Part model, mm, in its own coordinate system. A direction names the side the tool comes from. Give positions to 0.01 mm unless a question says otherwise; leave off trailing zeros. Write each loop counter-clockwise with the first axis right and the second up, starting at its lowest first coordinate (ties: lowest second). Pieces come first, ordered by that corner, then holes. Notation, with made-up numbers: M 79.5,48.5 L 96.5,48.5 A33 ccw 96.5,82.5 Z; hole C -20,25.25 d1. An arc over 180 degrees is marked long. Answer as CSV lines item,"result". Start each with the question number.
Item 1: Band-saw the part on C-C, the plane z = -8. List the corners of the cut face in (x, y), then the cut area to 3 significant figures.
Item 2: Pin check, flat tips, straight feed: pin 1 (5 mm diameter, centred on x = 7, z = 5, fed in from +Y); pin 2 (8 mm diameter, centred on x = 7, y = 11.8, fed in from +Z). Stop position of each tip, or through.
Item 3: Wall check: L1, parallel to Y at x = 7, z = -16.25; L2, parallel to Y at x = 8, z = 3; L3, parallel to Z at x = 11.5, y = 8. Give the ranges that are in metal, low to high. Write a range as from..to.
Item 4: Band-saw the part on D-D, the plane x = 13. List the corners of the cut face in (y, z), then the cut area to 3 significant figures.
Item 5: 3-axis set-ups, long thin cutter, end or side, ignore diameter. For faces 5 (the flat face through (7, 20, -15.506)), 6 (the cylindrical face through (8.61, 33.83, -16.49)): which of +Z, -Z, +X, -X, +Y, -Y reach the whole face in a straight line?
Item 6: Two-plate mould, pull along X, no slides. Class faces 1 (the flat face through (14, 1, -7)), 2 (the cylindrical face through (5.851, 1.014, 16.565)), 3 (the flat face through (0, 1, -7)), 4 (the flat face through (7, 0, 2)): +X half, -X half, draft (parallel to the pull), parting line (faces both ways), or undercut.
Item 7: Band-saw the part on B-B, the plane y = 29.5. List the corners of the cut face in (x, z), then the cut area to 3 significant figures.
Item 8: Band-saw the part on A-A, the plane x = 7. List the corners of the cut face in (y, z).
from build123d import *

# Parameters (mm, degrees)
BOSS_EXTRUDE1_DEPTH = 14
SKETCH2_R           = 3
CUT_EXTRUDE1_DEPTH  = 46.02225292
SKETCH3_R           = 3
CUT_EXTRUDE2_DEPTH  = 56.551777649


with BuildPart() as part:
    # Sketch1 → Boss-Extrude1 (new body)
    with BuildSketch(Plane(origin=(0, 0, 0), x_dir=(0, 0, -1), z_dir=(1, 0, 0))):
        Polygon((-21.494261048, 2), (15.505738952, 2), (15.505738952, 39), (17.505738952, 39), (17.505738952, 0), (-21.494261048, 0), align=None)
    extrude(amount=BOSS_EXTRUDE1_DEPTH)

    # Sketch2 → Cut-Extrude1 (cut, through all)
    with BuildSketch(Plane(origin=(0, 2, 0), x_dir=(1, 0, 0), z_dir=(0, 1, 0))):
        with Locations(Location((7, -13.794261048, 0), (0, 0, 270))):
            Circle(SKETCH2_R)
        with Locations(Location((7, 5.705738952, 0), (0, 0, 270))):
            Circle(SKETCH2_R)
    extrude(amount=-CUT_EXTRUDE1_DEPTH, mode=Mode.SUBTRACT)

    # Sketch3 → Cut-Extrude2 (cut, through all)
    with BuildSketch(Plane.XY.offset(-15.505738952)):
        with Locations((7, 11.8)):
            Circle(SKETCH3_R)
        with Locations((7, 31.3)):
            Circle(SKETCH3_R)
    extrude(amount=-CUT_EXTRUDE2_DEPTH, mode=Mode.SUBTRACT)


solid = part.part
Output:
1,outline,"M 0,0 L 5.07,0 L 5.07,2 L 0,2 Z; M 8.93,0 L 14,0 L 14,2 L 8.93,2 Z"
1,area,"20.3 mm²"
2,pin 1,"y = 2"
2,pin 2,"z = -15.51"
3,L1,"0..8.8, 14.8..28.3, 34.3..39"
3,L2,"0..2"
3,L3,"-17.51..-15.51"
4,outline,"M 0,-17.51 L 39,-17.51 L 39,-15.51 L 2,-15.51 L 2,21.49 L 0,21.49 Z"
4,area,"152 mm²"
5,face 5,"+Z, +X, -X, +Y"
5,face 6,"+Z, -Z"
6,face 1,"+X half"
6,face 2,"undercut"
6,face 3,"-X half"
6,face 4,"draft"
7,outline,"M 0,-17.51 L 4.6,-17.51 L 4.6,-15.51 L 0,-15.51 Z; M 9.4,-17.51 L 14,-17.51 L 14,-15.51 L 9.4,-15.51 Z"
7,area,"18.4 mm²"
8,outline,"M 0,-17.51 L 8.8,-17.51 L 8.8,-15.51 L 2,-15.51 L 2,-8.71 L 0,-8.71 Z; M 0,-2.71 L 2,-2.71 L 2,10.79 L 0,10.79 Z; M 0,16.79 L 2,16.79 L 2,21.49 L 0,21.49 Z; M 14.8,-17.51 L 28.3,-17.51 L 28.3,-15.51 L 14.8,-15.51 Z; M 34.3,-17.51 L 39,-17.51 L 39,-15.51 L 34.3,-15.51 Z"
